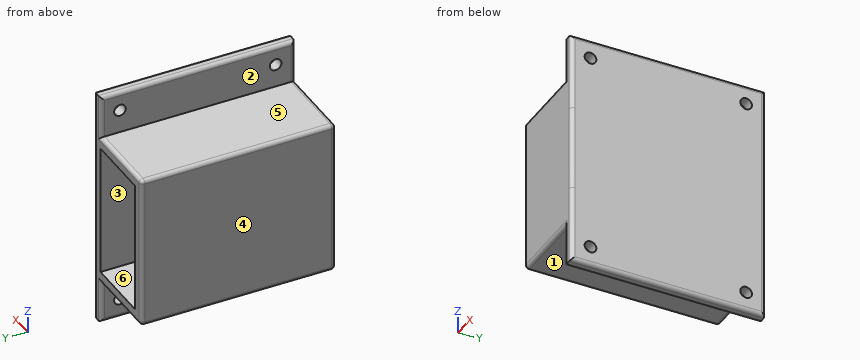
```python
from build123d import *

# Parameters (mm, degrees)
CROQUIS2_W              = 23
CROQUIS2_H              = 40
SALIENTE_EXTRUIR1_DEPTH = 50
CROQUIS3_W              = 17
CROQUIS3_H              = 34
CORTAR_EXTRUIR1_DEPTH   = 45
REDONDEO1_R             = 1
CROQUIS5_W              = 20
CROQUIS5_H              = 50
CROQUIS5_R              = 1.5
SALIENTE_EXTRUIR3_DEPTH = 3
REDONDEO2_R             = 1


with BuildPart() as part:
    # Croquis2 → Saliente-Extruir1 (new body)
    with BuildSketch(Plane(origin=(0, 0, 0), x_dir=(1, 0, 0), z_dir=(0, 1, 0))):
        with Locations((-11.5, 20)):
            Rectangle(CROQUIS2_W, CROQUIS2_H)
    extrude(amount=SALIENTE_EXTRUIR1_DEPTH)

    # Croquis3 → Cortar-Extruir1 (cut)
    with BuildSketch(Plane(origin=(0, 50, 0), x_dir=(1, 0, 0), z_dir=(0, 1, 0))):
        with Locations((-11.5, 20)):
            Rectangle(CROQUIS3_W, CROQUIS3_H)
    extrude(amount=-CORTAR_EXTRUIR1_DEPTH, mode=Mode.SUBTRACT)

    # Redondeo1
    redondeo1_edges = [part.edges().sort_by_distance(p)[0] for p in [
        (-11.5, 0, 0),
        (-23, 0, -20),
        (-11.5, 0, -40),
        (0, 0, -20),
        (0, 25, 0),
        (-23, 25, 0),
        (-23, 25, -40),
        (0, 25, -40),
    ]]
    fillet(redondeo1_edges, radius=REDONDEO1_R)

    # Croquis5 → Saliente-Extruir3 (add)
    # profile 1 of 2: a face of its own
    with BuildSketch(Plane(origin=(0, 0, 0), x_dir=(0, 0, -1), z_dir=(1, 0, 0))):
        with Locations((-1, 25)):
            Rectangle(CROQUIS5_W, CROQUIS5_H)
        with Locations((-6, 45)):
            Circle(CROQUIS5_R, mode=Mode.SUBTRACT)
        with Locations((-6, 5)):
            Circle(CROQUIS5_R, mode=Mode.SUBTRACT)
    # profile 2 of 2: a face of its own
    with BuildSketch(Plane(origin=(0, 0, 0), x_dir=(0, 0, -1), z_dir=(1, 0, 0))):
        with Locations((41, 25)):
            Rectangle(CROQUIS5_W, CROQUIS5_H)
        with Locations((46, 5)):
            Circle(CROQUIS5_R, mode=Mode.SUBTRACT)
        with Locations((46, 45)):
            Circle(CROQUIS5_R, mode=Mode.SUBTRACT)
    extrude(amount=-SALIENTE_EXTRUIR3_DEPTH)

    # Redondeo2
    redondeo2_edges = [part.edges().sort_by_distance(p)[0] for p in [
        (-12.5, 50, 0),
        (-22.707106781, 50, -0.292893219),
        (-23, 50, -20),
        (-22.707106781, 50, -39.707106781),
        (-12.5, 50, -40),
        (-3, 0, -45),
        (-3, 25, -51),
        (-3, 50, -45.5),
        (0, 25, -51),
        (0, 0, -41),
        (0, 0, 1),
        (0, 25, 11),
        (-3, 25, 11),
        (0, 50, -20),
        (-3, 50, 5.5),
        (-3, 0, 5),
    ]]
    fillet(redondeo2_edges, radius=REDONDEO2_R)


solid = part.part
```
Geometry check sheet. Reference: the model listing, model coordinates, mm. Face numbers are marked on the shaded views. A direction names the side the tool comes from. Give positions to 0.01 mm unless a question says otherwise; leave off trailing zeros. Order: outer loops, then holes, each group sorted by start corner. A loop starts at its lowest first (then second) coordinate and runs counter-clockwise, first axis right, second up. Notation, with made-up numbers: (10.5, 36) - (28.5, 36) arc R19 cw to (28.5, 58) - close; hole circle Ø8 at (-26.5, 0.5). An arc over 180 degrees is marked (long way). Answer in a Markdown table with one row per item. Add a question column.
Q1. Cross-section at C-C, the plane y = 14. Enter the section's corners in (x, z).
Q2. Cross-section at A-A, the plane y = 45. Enter the section's corners in (x, z), then the cut area to 3 significant figures.
Q3. Mould release check, pull along Z, two halves, no side actions. Record for the marked faces 4, 5 and 6: pulls with the +Z half, pulls with the -Z half, needs draft (parallel to the pull), parting line crosses it, or undercut.
Q4. Cross-section at B-B, the plane z = 6. Enter the section's corners in (x, y).
Q5. Material ranges on probe 1 along Y at (x, z) = (-1.45, 6); probe 2 along X at (y, z) = (18, -23); probe 3 along Z at (x, y) = (-15.5, 14.5), recorded low to high. Write a range as from..to.
Q6. Cross-section at D-D, the plane z = -8. Enter the section's corners in (x, y).
Q7. Gauge pin test, flat ends, axial feed: pin 1 (1.5 mm diameter, centred on x = -8, z = -30.5, fed in from +Y); pin 2 (1.8 mm diameter, centred on y = 5, z = 6, fed in from +X); pin 3 (5 mm diameter, centred on x = -14.5, y = 18, fed in from -Z); pin 4 (2 mm diameter, centred on x = -9, y = 41.5, fed in from +Z). Record the tip position at first contact, or that the pin passes through.
Q8. Tool access check on the marked faces 1, 2 and 3. Record the directions out of +Z, -Z, +X, -X, +Y, -Y that give a thin tool (end or side, any length) a straight path to the whole face; none if there is none.
Check values:
| question | item | result |
|---|---|---|
| 1 | outline | (-23, -39) arc R1 ccw to (-22, -40) - (-3, -40) - (-3, -50) arc R1 ccw to (-2, -51) - (-1, -51) arc R1 ccw to (0, -50) - (0, 10) arc R1 ccw to (-1, 11) - (-2, 11) arc R1 ccw to (-3, 10) - (-3, 0) - (-22, 0) arc R1 ccw to (-23, -1) - close; hole (-20, -37) - (-3, -37) - (-3, -3) - (-20, -3) - close |
| 2 | outline | (-23, -39) arc R1 ccw to (-22, -40) - (-3, -40) - (-3, -44.5) - (0, -44.5) - (0, 4.5) - (-3, 4.5) - (-3, 0) - (-22, 0) arc R1 ccw to (-23, -1) - close; (-3, -50) arc R1 ccw to (-2, -51) - (-1, -51) arc R1 ccw to (0, -50) - (0, -47.5) - (-3, -47.5) - close; (-3, 7.5) - (0, 7.5) - (0, 10) arc R1 ccw to (-1, 11) - (-2, 11) arc R1 ccw to (-3, 10) - close; hole (-20, -37) - (-3, -37) - (-3, -3) - (-20, -3) - close |
| 2 | area | 389 mm^2 |
| 3 | face 4 | needs draft |
| 3 | face 5 | pulls with the +Z half |
| 3 | face 6 | undercut |
| 4 | outline | (-3, 1) arc R1 ccw to (-2, 0) - (-1, 0) arc R1 ccw to (0, 1) - (0, 3.5) - (-3, 3.5) - close; (-3, 6.5) - (0, 6.5) - (0, 43.5) - (-3, 43.5) - close; (-3, 46.5) - (0, 46.5) - (0, 49) arc R1 ccw to (-1, 50) - (-2, 50) arc R1 ccw to (-3, 49) - close |
| 5 | probe 1 | y = 0..3.5, 6.5..43.5, 46.5..50 |
| 5 | probe 2 | x = -23..-20, -3..0 |
| 5 | probe 3 | z = -40..-37, -3..0 |
| 6 | outline | (-23, 1) arc R1 ccw to (-22, 0) - (-1, 0) arc R1 ccw to (0, 1) - (0, 49) arc R1 ccw to (-1, 50) - (-3, 50) - (-3, 5) - (-20, 5) - (-20, 50) - (-22, 50) arc R1 ccw to (-23, 49) - close |
| 7 | pin 1 | stops at y = 5 |
| 7 | pin 2 | passes through |
| 7 | pin 3 | stops at z = -40 |
| 7 | pin 4 | stops at z = 0 |
| 8 | face 1 | -Z, -X, +Y, -Y |
| 8 | face 2 | +Z, -X, +Y, -Y |
| 8 | face 3 | +Y |
